from build123d import *

# Parameters (mm, degrees)
CROQUIS1_W                   = 200
CROQUIS1_H                   = 52.5
SALIENTE_EXTRUIR1_DEPTH      = 4.6
CROQUIS2_R                   = 7.05
CORTAR_EXTRUIR1_DEPTH        = 3.6
TALADRO_DE_MARGEN_PARA_M31_D = 3.4
CHAFL_N1_SIZE                = 3
TALADRO_DE_MARGEN_PARA_M32_D = 3.4
CORTAR_EXTRUIR2_DEPTH        = 104.490204851
TALADRO_DE_MARGEN_PARA_M33_D = 3.4
TALADRO_DE_MARGEN_PARA_M81_D = 9


with BuildPart() as part:
    # Croquis1 → Saliente-Extruir1 (new body)
    with BuildSketch(Plane(origin=(0, 0, 0), x_dir=(0, 1, 0), z_dir=(0, 0, 1))):
        Rectangle(CROQUIS1_W, CROQUIS1_H)
    extrude(amount=SALIENTE_EXTRUIR1_DEPTH)

    # Croquis2 → Cortar-Extruir1 (cut)
    with BuildSketch(Plane.XY.offset(4.6)):
        with Locations((12.5, -80)):
            Circle(CROQUIS2_R)
    extrude(amount=-CORTAR_EXTRUIR1_DEPTH, mode=Mode.SUBTRACT)

    # Taladro de margen para M31 (through all)
    with Locations(Plane(origin=(0, 0, 0), x_dir=(1, 0, 0), z_dir=(0, 0, -1))):
        with Locations((19.25, -45), (19.25, 45), (0.75, 45), (0.75, -45)):
            Hole(TALADRO_DE_MARGEN_PARA_M31_D / 2)

    # Chaflán1
    chafl_n1_edges = [part.edges().sort_by_distance(p)[0] for p in [
        (26.25, 100, 2.3),
        (26.25, -100, 2.3),
        (-26.25, -100, 2.3),
        (-26.25, 100, 2.3),
    ]]
    chamfer(chafl_n1_edges, length=CHAFL_N1_SIZE)

    # Taladro de margen para M32 (through all)
    with Locations(Plane.XY.offset(4.6)):
        with Locations((-22.75, -60), (-22.75, -40), (-22.75, 40), (-22.75, 60)):
            Hole(TALADRO_DE_MARGEN_PARA_M32_D / 2)

    # Croquis8 → Cortar-Extruir2 (cut, through all)
    with BuildSketch(Plane.XY.offset(4.6)):
        Polygon((-5.840411229, 33.2), (5.840411229, 33.2), (14.1, 24.940411229), (14.1, 13.259588771), (5.840411229, 5), (-5.840411229, 5), (-14.1, 13.259588771), (-14.1, 24.940411229), align=None)
        Polygon((5.840411229, -33.2), (14.1, -24.940411229), (14.1, -13.259588771), (5.840411229, -5), (-5.840411229, -5), (-14.1, -13.259588771), (-14.1, -24.940411229), (-5.840411229, -33.2), align=None)
        Polygon((13.297005384, -61), (7.523502692, -51), (-4.023502692, -51), (-9.797005384, -61), (-4.023502692, -71), (7.523502692, -71), align=None)
        Polygon((5.840411229, 56.8), (14.1, 65.059588771), (14.1, 76.740411229), (5.840411229, 85), (-5.840411229, 85), (-14.1, 76.740411229), (-14.1, 65.059588771), (-5.840411229, 56.8), align=None)
    extrude(amount=-CORTAR_EXTRUIR2_DEPTH, mode=Mode.SUBTRACT)

    # Taladro de margen para M33 (through all)
    with Locations(Plane.XY.offset(4.6)):
        with Locations((0.75, 92.5), (19.25, 92.5)):
            Hole(TALADRO_DE_MARGEN_PARA_M33_D / 2)

    # Taladro de margen para M81 (through all)
    with Locations(Plane(origin=(0, 0, 0), x_dir=(1, 0, 0), z_dir=(0, 0, -1))):
        with Locations((-11.5, 69.7), (-11.5, 90.3)):
            Hole(TALADRO_DE_MARGEN_PARA_M81_D / 2)


solid = part.part
Build history of the part. All positions in model axes, mm. A direction names the side the tool comes from. Coordinates: 2 decimals unless noted, no trailing zeros. Write each loop counter-clockwise with the first axis right and the second up, starting at its lowest first coordinate (ties: lowest second). Pieces come first, ordered by that corner, then holes.
(1) Cut at D-D on y = -68. List the corners of the cut face in (x, z), and give its area (3 significant figures).
(2) Cut at B-B on x = 0.75. State how many separate pieces and enclosed holes the cut face has, and give its area (3 significant figures).
(3) Mould opens along Y. For faces 1 (the flat face through (26.25, -1, 2)), 2 (the flat face through (14.1, 71, 2)), 3 (the flat face through (0, 100, 2)) say: pulls with the +Y half, pulls with the -Y half, needs draft (parallel to the pull), parting line crosses it, or undercut.
(4) Cut at C-C on x = -12. List the corners of the cut face in (y, z).
(5) 3-axis set-ups, long thin cutter, end or side, ignore diameter. For faces 4 (the flat face through (-14.1, -19, 2)), 5 (the cylindrical face through (11.58, -73.01, 2.83)), 6 (the flat face through (0, -1, 0)): which of +Z, -Z, +X, -X, +Y, -Y reach the whole face in a straight line?
(6) Drill centre lines: line 1 (X direction, y = 45, z = 3.4); line 2 (Y direction, x = -22.75, z = 2.35); line 3 (Y direction, x = -3, z = 2.85). Where is each one in solid material? Low to high.
(7) Cut at A-A on y = -40. List the corners of the cut face in (x, z).
(8) Pin check, flat tip, straight feed: pin 1 Ø2 at (x, y) = (0.75, 92.5) entering from +Z. Stop position of the tip, or through.
Working result:
1. outline: (-26.25, 0) - (-15.67, 0) - (-15.67, 4.6) - (-26.25, 4.6) - close; (-7.33, 0) - (-5.76, 0) - (-5.76, 4.6) - (-7.33, 4.6) - close; (9.26, 0) - (26.25, 0) - (26.25, 4.6) - (9.26, 4.6) - close
1. area: 134 mm2
2. separate pieces: 8
2. enclosed holes: 0
2. area: 392 mm2
3. face 1: needs draft
3. face 2: undercut
3. face 3: pulls with the +Y half
4. outline: (-100, 0) - (-94.77, 0) - (-94.77, 4.6) - (-100, 4.6) - close; (-85.83, 0) - (-74.17, 0) - (-74.17, 4.6) - (-85.83, 4.6) - close; (-65.23, 0) - (-27.04, 0) - (-27.04, 4.6) - (-65.23, 4.6) - close; (-11.16, 0) - (11.16, 0) - (11.16, 4.6) - (-11.16, 4.6) - close; (27.04, 0) - (62.96, 0) - (62.96, 4.6) - (27.04, 4.6) - close; (78.84, 0) - (100, 0) - (100, 4.6) - (78.84, 4.6) - close
5. face 4: +Z, -Z
5. face 5: +Z
5. face 6: -Z, +X, -X, +Y, -Y
6. line 1: x = -26.25 to -0.95, 2.45 to 17.55, 20.95 to 26.25
6. line 2: y = -100 to -61.7, -58.3 to -41.7, -38.3 to 38.3, 41.7 to 58.3, 61.7 to 100
6. line 3: y = -100 to -71, -51 to -33.2, -5 to 5, 33.2 to 56.8, 85 to 100
7. outline: (-26.25, 0) - (-24.45, 0) - (-24.45, 4.6) - (-26.25, 4.6) - close; (-21.05, 0) - (26.25, 0) - (26.25, 4.6) - (-21.05, 4.6) - close
8. pin 1: passes through
